Build history of the part. All positions in model axes, mm. A direction names the side the tool comes from. Give positions to 0.01 mm unless a question says otherwise; leave off trailing zeros. Order: outer loops, then holes, each group sorted by start corner. A loop starts at its lowest first (then second) coordinate and runs counter-clockwise, first axis right, second up. Notation, with made-up numbers: (75.25, 88.25) - (119.25, 88.25) arc R25 ccw to (119.25, 123.25) - close; hole circle Ø9 at (88.5, 31.5). An arc over 180 degrees is marked (long way). Answer in a Markdown table with one row per item.
```python
from build123d import *

# Parameters (mm, degrees)
CUT_EXTRUDE_1_REACH = 16.841
SKETCH_2_R          = 1.5


with BuildPart() as part:
    # 草图1 → 旋转1 (revolve)
    with BuildSketch(Plane.XY, mode=Mode.PRIVATE) as revolve_1_sk:
        Polygon((0, 4.5), (-10, 4.5), (-10, 2.5), (-4.5, 2.5), (-4.5, 0), (-2.75, 0), (-2.75, 3.5), (0, 3.5), align=None)
    revolve(revolve_1_sk.sketch.rotate(Axis((0, 0, 0), (0, 1, 0)), 270), axis=Axis((0, 0, 0), (0, 1, 0)))

    # 草图2 → 切除-拉伸1 (cut, up to next)
    with BuildSketch(Plane(origin=(0, 4.5, 0), x_dir=(1, 0, 0), z_dir=(0, 1, 0)), mode=Mode.PRIVATE) as cut_extrude_1_sk1:
        with Locations(Location((0, 7, 0), (0, 0, 270))):
            Circle(SKETCH_2_R)
    cut_extrude_1_tool1 = extrude(cut_extrude_1_sk1.sketch, amount=-CUT_EXTRUDE_1_REACH, mode=Mode.PRIVATE) & part.part
    # 草图2 → 切除-拉伸1 (cut, up to next)
    with BuildSketch(Plane(origin=(0, 4.5, 0), x_dir=(1, 0, 0), z_dir=(0, 1, 0)), mode=Mode.PRIVATE) as cut_extrude_1_sk2:
        with Locations(Location((7, 0, 0), (0, 0, 270))):
            Circle(SKETCH_2_R)
    cut_extrude_1_tool2 = extrude(cut_extrude_1_sk2.sketch, amount=-CUT_EXTRUDE_1_REACH, mode=Mode.PRIVATE) & part.part
    # 草图2 → 切除-拉伸1 (cut, up to next)
    with BuildSketch(Plane(origin=(0, 4.5, 0), x_dir=(1, 0, 0), z_dir=(0, 1, 0)), mode=Mode.PRIVATE) as cut_extrude_1_sk3:
        with Locations(Location((0, -7, 0), (0, 0, 270))):
            Circle(SKETCH_2_R)
    cut_extrude_1_tool3 = extrude(cut_extrude_1_sk3.sketch, amount=-CUT_EXTRUDE_1_REACH, mode=Mode.PRIVATE) & part.part
    # 草图2 → 切除-拉伸1 (cut, up to next)
    with BuildSketch(Plane(origin=(0, 4.5, 0), x_dir=(1, 0, 0), z_dir=(0, 1, 0)), mode=Mode.PRIVATE) as cut_extrude_1_sk4:
        with Locations(Location((-7, 0, 0), (0, 0, 270))):
            Circle(SKETCH_2_R)
    cut_extrude_1_tool4 = extrude(cut_extrude_1_sk4.sketch, amount=-CUT_EXTRUDE_1_REACH, mode=Mode.PRIVATE) & part.part
    add(cut_extrude_1_tool1.solids().sort_by_distance((0, 4.5, -7))[0], mode=Mode.SUBTRACT)
    add(cut_extrude_1_tool2.solids().sort_by_distance((7, 4.5, 0))[0], mode=Mode.SUBTRACT)
    add(cut_extrude_1_tool3.solids().sort_by_distance((0, 4.5, 7))[0], mode=Mode.SUBTRACT)
    add(cut_extrude_1_tool4.solids().sort_by_distance((-7, 4.5, 0))[0], mode=Mode.SUBTRACT)


solid = part.part
```
1. Cut at B-B on z = 0. Write the cut outline in (x, y).
Check result:
| item | result |
|---|---|
| outline | (-10, 2.5) - (-8.5, 2.5) - (-8.5, 4.5) - (-10, 4.5) - close; (-5.5, 2.5) - (-4.5, 2.5) - (-4.5, 0) - (-2.75, 0) - (-2.75, 3.5) - (2.75, 3.5) - (2.75, 0) - (4.5, 0) - (4.5, 2.5) - (5.5, 2.5) - (5.5, 4.5) - (-5.5, 4.5) - close; (8.5, 2.5) - (10, 2.5) - (10, 4.5) - (8.5, 4.5) - close |
2. Which spindle directions (+Z, -Z, +X, -X, +Y, -Y) get a long thin tool onto all of the face, cutting with end or side? Do faces 4 (the face through (5.536, 3.514, -0.325)), 5 (the face through (2.1, 2.5, -4.3)). Say none if no direction does.
Check result:
| item | result |
|---|---|
| face 4 | +Y, -Y |
| face 5 | -Y |
3. Cut at A-A on x = 0. Write the cut outline in (y, z).
Check result:
| item | result |
|---|---|
| outline | (0, -4.5) - (2.5, -4.5) - (2.5, -5.5) - (4.5, -5.5) - (4.5, 5.5) - (2.5, 5.5) - (2.5, 4.5) - (0, 4.5) - (0, 2.75) - (3.5, 2.75) - (3.5, -2.75) - (0, -2.75) - close; (2.5, -10) - (4.5, -10) - (4.5, -8.5) - (2.5, -8.5) - close; (2.5, 8.5) - (4.5, 8.5) - (4.5, 10) - (2.5, 10) - close |
4. Cut at D-D on z = -7. Write the cut outline in (x, y), and give its area (3 significant figures).
Check result:
| item | result |
|---|---|
| outline | (-7.14, 2.5) - (-1.5, 2.5) - (-1.5, 4.5) - (-7.14, 4.5) - close; (1.5, 2.5) - (7.14, 2.5) - (7.14, 4.5) - (1.5, 4.5) - close |
| area | 22.6 mm² |
5. Cut at C-C on y = 3.85. Write the cut outline in (x, z), and give its area (3 significant figures).
Check result:
| item | result |
|---|---|
| outline | circle Ø20 at (0, 0); hole circle Ø3 at (-7, 0); hole circle Ø3 at (0, -7); hole circle Ø3 at (0, 7); hole circle Ø3 at (7, 0) |
| area | 286 mm² |
6. Drop flat-ended pins along their axis: P1, Ø1.5, axis at x = -3, z = -7.5, coming from the -Y side; P2, Ø1, axis at y = 0.5, z = 2.5, coming from the -X side. Give the stop position or say it passes through.
Check result:
| item | result |
|---|---|
| P1 | stops at y = 2.5 |
| P2 | stops at x = -4.03 |
7. Probe line 1 (X direction, y = 3.6, z = 0); line 2 (Y direction, x = -7.5, z = 3.75); line 3 (Z direction, x = -1.25, y = 3). List the from-to ranges inside material, lowest first.
Check result:
| item | result |
|---|---|
| line 1 | x = -10 to -8.5, -5.5 to 5.5, 8.5 to 10 |
| line 2 | y = 2.5 to 4.5 |
| line 3 | z = -9.92 to -7.83, -6.17 to -2.45, 2.45 to 6.17, 7.83 to 9.92 |
8. Two-plate mould, pull along Z, no slides. Class faces 1 (the face through (0.07, 3.51, 5.5)), 2 (the face through (0, 4.5, 0)), 3 (the face through (-1.352, 1.232, -4.292)): +Z half, -Z half, draft (parallel to the pull), parting line (faces both ways), or undercut.
Check result:
| item | result |
|---|---|
| face 1 | undercut |
| face 2 | draft |
| face 3 | parting line |
